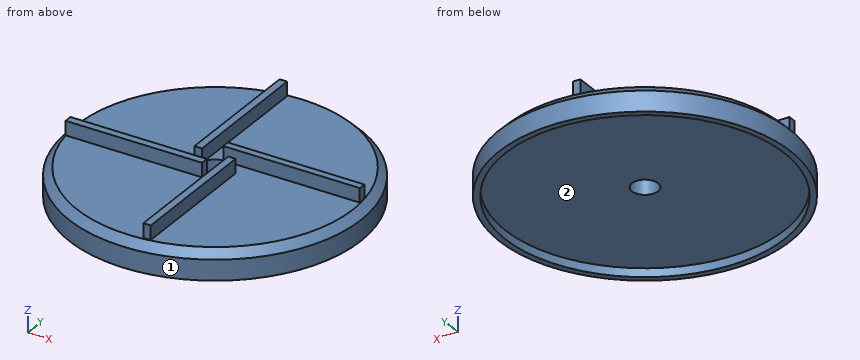
```python
from build123d import *

# Parameters (mm, degrees)
F0_R     = 47.0892297355
F0_R_2   = 45.1105774951
F0_R_3   = 10.9409208949
F0_R_4   = 4.2395211019
F1_DEPTH = 3.81
F2_SIZE  = 2.54
F3_R     = 47.0892297355
F3_R_2   = 45.1105774951
F4_DEPTH = 5.334
F6_DEPTH = 2.54
F5_W     = 2.4396785341
F5_H     = 43.9290553331
F5_W_2   = 44.0566511325
F5_H_2   = 2.3669424772
F5_W_3   = 2.3844161808
F5_H_3   = 43.7675852008
F5_W_4   = 44.0356882348
F5_H_4   = 2.5052570053
F7_DEPTH = 4.572


with BuildPart() as f1:
    # F0 (on Top) → F1 (new body)
    with BuildSketch(Plane.XY):
        Circle(F0_R)
        Circle(F0_R_2, mode=Mode.SUBTRACT)
        Circle(F0_R_2)
        Circle(F0_R_3, mode=Mode.SUBTRACT)
        Circle(F0_R_3)
        Circle(F0_R_4, mode=Mode.SUBTRACT)
    extrude(amount=F1_DEPTH)

    # F2
    f2_edges = [f1.edges().sort_by_distance(p)[0] for p in [
        (-47.08923, 0, 3.81),
    ]]
    chamfer(f2_edges, length=F2_SIZE)

    # F3 (on face) → F4 (join)
    with BuildSketch(Plane(origin=(0, 0, 0), x_dir=(1, 0, 0), z_dir=(0, 0, -1))):
        Circle(F3_R)
        Circle(F3_R_2, mode=Mode.SUBTRACT)
    extrude(amount=F4_DEPTH)

    # F6 (add): a face of the model
    f6_faces = [f1.faces().sort_by_distance(p)[0] for p in [
        (-43.8346576851, 0, 0),
    ]]
    extrude(f6_faces, amount=F6_DEPTH)

    # F5 (on face) → F7 (join)
    with BuildSketch(Plane.XY.offset(3.81)):
        with Locations((-5.4593603689, 21.9645276666)):
            Rectangle(F5_W, F5_H)
        with Locations((22.0283255662, 5.4229923405)):
            Rectangle(F5_W_2, F5_H_2)
        with Locations((5.4317291923, -21.8837926004)):
            Rectangle(F5_W_3, F5_H_3)
        with Locations((-22.0178441174, -5.4921496045)):
            Rectangle(F5_W_4, F5_H_4)
    extrude(amount=F7_DEPTH)


solid = f1.part
```
For this review, take the finished solid that the model builds, in its own axes (mm). Face numbers are marked on the shaded views. Round coordinates to 2 decimals unless told otherwise and drop trailing zeros. Write each loop counter-clockwise with the first axis right and the second up, starting at its lowest first coordinate (ties: lowest second). Pieces come first, ordered by that corner, then holes. Notation, with made-up numbers: (-35, 7) - (9, 7) arc R24 cw to (9, 17) - close; hole circle Ø11 at (-17, -21.5). An arc over 180 degrees is marked (long way). Write each question's results on one line, items separated by ' | '.
Item 1: Take a section at A-A on z = 6.75. State the section outline as (x, y) points.
Calculated:
outline: (-44.04, -6.74) - (0, -6.74) - (0, -4.24) - (-44.04, -4.24) - close; (-6.68, 0) - (-4.24, 0) - (-4.24, 43.93) - (-6.68, 43.93) - close; (0, 4.24) - (44.06, 4.24) - (44.06, 6.61) - (0, 6.61) - close; (4.24, -43.77) - (6.62, -43.77) - (6.62, 0) - (4.24, 0) - close
Item 2: For pin 1 (2.5 mm diameter, centred on y = 5.5, z = 5, fed in from +X); pin 2 (2 mm diameter, centred on x = -29.5, y = -18, fed in from +Z); pin 3 (0.7 mm diameter, centred on x = 5, z = 6.5, fed in from -Y), all flat-tipped, find the tip position at first contact; note any pin that passes through.
Calculated:
pin 1: stops at x = 44.28 | pin 2: stops at z = 3.81 | pin 3: stops at y = -43.77
Item 3: Draft analysis for pull direction X (two halves, no side actions). For the marked faces 1 and 2, state which applies: pulls with the +X half, pulls with the -X half, needs draft (parallel to the pull), parting line crosses it, or undercut.
Calculated:
face 1: parting line crosses it | face 2: undercut
Item 4: To check wall thickness, follow line 1 along Y through (x, z) = (0, -4.2); line 2 along Y through (x, z) = (0, 0); line 3 along Y through (x, z) = (-38, 6.5). State the ranges of each line that lie inside material, in increasing order. Write a range as from..to.
Calculated:
line 1: y = -47.09..-45.11, 45.11..47.09 | line 2: y = -47.09..-4.24, 4.24..47.09 | line 3: y = -6.74..-4.24
